The model under review builds one solid part; all positions refer to its coordinate system, in mm. A direction names the side the tool comes from. Round coordinates to 2 decimals unless told otherwise and drop trailing zeros. Loops run counter-clockwise (first coordinate to the right, second up) from the corner with the lowest first, then second, coordinate; pieces in that order, holes last. Notation, with made-up numbers: (74, 80) -> (116, 80) arc R3 cw to (116, 84) -> close; hole circle Ø5 at (-35, -31). An arc over 180 degrees is marked (long way). Return JSON: item names as keys, results as strings. Group by question number.
```python
from build123d import *

# Parameters (mm, degrees)
BOSS_EXTRUDE1_DEPTH = 1.524


with BuildPart() as part:
    # Sketch1 → Boss-Extrude1 (new body)
    with BuildSketch(Plane.XY):
        with BuildLine():
            Line((41.68481024, 0), (41.68481024, -1.524))
            Line((41.68481024, -1.524), (36.357969238, -1.524))
            ThreePointArc((36.357969238, -1.524), (40.575187599, -6.520629639), (47.11110588, -6.702318062))
            ThreePointArc((47.11110588, -6.702318062), (48.381195539, -5.722313338), (49.840736605, -5.056522921))
            ThreePointArc((49.840736605, -5.056522921), (45.764525456, -4.822424484), (41.860759392, -3.626218014))
            Line((41.860759392, -3.626218014), (41.860759392, -2.667580322))
            Line((41.860759392, -2.667580322), (46.80618972, -1.524))
            Line((46.80618972, -1.524), (46.80618972, 0))
            Line((46.80618972, 0), (41.860759392, 1.143580322))
            Line((41.860759392, 1.143580322), (41.860759392, 2.102218014))
            ThreePointArc((41.860759392, 2.102218014), (45.764525456, 3.298424484), (49.840736605, 3.532522921))
            ThreePointArc((49.840736605, 3.532522921), (48.381195539, 4.198313338), (47.11110588, 5.178318062))
            ThreePointArc((47.11110588, 5.178318062), (42.874226953, 5.702520491), (38.97108533, 3.972949241))
            Line((38.97108533, 3.972949241), (39.021389739, 0))
            Line((39.021389739, 0), (41.68481024, 0))
        make_face()
    extrude(amount=BOSS_EXTRUDE1_DEPTH)


solid = part.part
```
1. We need section A-A, the plane x = 42.5. Write out the cut boundary in (y, z).
2. For P1, Ø0.8, axis at y = -0.5, z = 1, coming from the +X side; P2, Ø0.5, axis at x = 41, z = 0.5, coming from the -Y side; P3, Ø0.5, axis at y = -1, z = 0.5, coming from the -X side, all flat-tipped, find the tip position at first contact; note any pin that passes through.
3. Tool access review of faces 5 (the face through (41.685, -1, 1)), 6 (the face through (48.362, -5.734, 0.751)), 7 (the face through (44.368, 0.564, 0.751)): name each direction out of +Z, -Z, +X, -X, +Y, -Y from which nothing blocks a thin tool from reaching the whole face with its end or side.
4. We need section C-C, the plane x = 39.75. Write out the cut boundary in (y, z).
5. We need section D-D, the plane y = -0.25. Write out the cut boundary in (x, z).
6. Wall thickness on line 1 (Y direction, x = 46, z = 0.85); line 2 (Y direction, x = 42, z = 1.4); line 3 (X direction, y = -0.75, z = 0.9): over which ranges is each line inside the solid? List them lowest first.
7. Draft analysis for pull direction X (two halves, no side actions). For faces 1 (the face through (39, -1.524, 1)), 2 (the face through (45.71, 3.29, 0.75)), 3 (the face through (46.806, -1, 1)), 4 (the face through (45.821, -4.832, 0.751)), state which applies: pulls with the +X half, pulls with the -X half, needs draft (parallel to the pull), parting line crosses it, or undercut.
8. We need section B-B, the plane z = 0.2. Write out the cut boundary in (x, y).
Check sheet entries:
{
 "1": {"outline": "(-7.16, 0) -> (-3.89, 0) -> (-3.89, 1.52) -> (-7.16, 1.52) -> close; (-2.52, 0) -> (1, 0) -> (1, 1.52) -> (-2.52, 1.52) -> close; (2.37, 0) -> (5.64, 0) -> (5.64, 1.52) -> (2.37, 1.52) -> close"},
 "2": {"P1": "stops at x = 46.81", "P2": "stops at y = -6.81", "P3": "stops at x = 41.68"},
 "3": {"face 5": "+Z, -Z, -X", "face 6": "+Z, -Z, +X, -Y", "face 7": "+Z, -Z, +X"},
 "4": {"outline": "(-6.06, 0) -> (-1.52, 0) -> (-1.52, 1.52) -> (-6.06, 1.52) -> close; (0, 0) -> (4.54, 0) -> (4.54, 1.52) -> (0, 1.52) -> close"},
 "5": {"outline": "(41.68, 0) -> (46.81, 0) -> (46.81, 1.52) -> (41.68, 1.52) -> close"},
 "6": {"line 1": "y = -7.07 to -4.86, -1.71 to 0.19, 3.34 to 5.55", "line 2": "y = -7.05 to -3.69, -2.64 to 1.11, 2.16 to 5.52", "line 3": "x = 41.68 to 46.81"},
 "7": {"face 1": "needs draft", "face 2": "undercut", "face 3": "pulls with the +X half", "face 4": "undercut"},
 "8": {"outline": "(36.36, -1.52) arc R8 ccw to (47.11, -6.7) arc R7.01 cw to (49.84, -5.06) arc R17.06 cw to (41.86, -3.63) -> (41.86, -2.67) -> (46.81, -1.52) -> (46.81, 0) -> (41.86, 1.14) -> (41.86, 2.1) arc R17.06 cw to (49.84, 3.53) arc R7.01 cw to (47.11, 5.18) arc R8 ccw to (38.97, 3.97) -> (39.02, 0) -> (41.68, 0) -> (41.68, -1.52) -> close"}
}
